Geometry: final body of the model. Coordinates: model frame, mm. Coordinates: 2 decimals unless noted, no trailing zeros. Order: outer loops, then holes, each group sorted by start corner. A loop starts at its lowest first (then second) coordinate and runs counter-clockwise, first axis right, second up. Notation, with made-up numbers: (-3, 76) - (33, 76) arc R26 cw to (33, 114) - close; hole circle Ø4 at (-29, -13.5). An arc over 180 degrees is marked (long way). Use a Markdown table: item, result. Add a question column.
```python
from build123d import *

# Parameters (mm, degrees)
SKETCH1_W            = 200
SKETCH1_H            = 114.3
BOSS_EXTRUDE1_DEPTH  = 6.8
SKETCH2_R            = 2.75
CUT_EXTRUDE1_DEPTH   = 6.8
FILLET1_R            = 3
FILLET1_OF_MIRROR2_R = 3


with BuildPart() as part:
    # Sketch1 → Boss-Extrude1 (new body)
    with BuildSketch(Plane.XY):
        Rectangle(SKETCH1_W, SKETCH1_H)
    extrude(amount=BOSS_EXTRUDE1_DEPTH)

    # Sketch2 → Cut-Extrude1 (cut)
    with BuildSketch(Plane.XY.offset(6.8)):
        with Locations((-92, 25.25)):
            Circle(SKETCH2_R)
    cut_extrude1 = extrude(amount=-CUT_EXTRUDE1_DEPTH, mode=Mode.SUBTRACT)

    # Fillet1
    fillet1_edges = [part.edges().sort_by_distance(p)[0] for p in [
        (-100, 57.15, 3.4),
        (-100, -57.15, 3.4),
    ]]
    fillet(fillet1_edges, radius=FILLET1_R)

    # Mirror2: Cut-Extrude1 across plane
    add(cut_extrude1.mirror(Plane(origin=(0, 0, 0), x_dir=(0, 0, 1), z_dir=(1, 0, 0))), mode=Mode.SUBTRACT)

    # Fillet1 of Mirror2
    fillet1_of_mirror2_edges = [part.edges().sort_by_distance(p)[0] for p in [
        (100, 57.15, 3.4),
        (100, -57.15, 3.4),
    ]]
    fillet(fillet1_of_mirror2_edges, radius=FILLET1_OF_MIRROR2_R)


solid = part.part
```
1) Section A-A (x = -92). Return loops of the section in (y, z), then the cut area to 3 significant figures.
2) Section B-B (y = 25.25). Return loops of the section in (x, z).
3) Pin query (flat end, axial travel): pin 1 (5 mm diameter, centred on x = 92, y = 25.25, fed in from -Z). Return the tip coordinate at first contact, or that it passes through.
4) Draft query along X for faces 1 (the face through (-1, 1, 6.8)), 2 (the face through (100, -1, 3)), 3 (the face through (-94.747, 25.371, 3.448)), 4 (the face through (-100, -1, 3)). Return one class per face: pulls with the +X half, pulls with the -X half, needs draft (parallel to the pull), parting line crosses it, or undercut.
5) Ray query, line 1 along Y through (x, z) = (92, 4). Return the intervals inside material, ascending.
Values follow:
| question | item | result |
|---|---|---|
| 1 | outline | (-57.15, 0) - (22.5, 0) - (22.5, 6.8) - (-57.15, 6.8) - close; (28, 0) - (57.15, 0) - (57.15, 6.8) - (28, 6.8) - close |
| 1 | area | 740 mm² |
| 2 | outline | (-100, 0) - (-94.75, 0) - (-94.75, 6.8) - (-100, 6.8) - close; (-89.25, 0) - (89.25, 0) - (89.25, 6.8) - (-89.25, 6.8) - close; (94.75, 0) - (100, 0) - (100, 6.8) - (94.75, 6.8) - close |
| 3 | pin 1 | passes through |
| 4 | face 1 | needs draft |
| 4 | face 2 | pulls with the +X half |
| 4 | face 3 | undercut |
| 4 | face 4 | pulls with the -X half |
| 5 | line 1 | y = -57.15 to 22.5, 28 to 57.15 |
